Part model, mm, in its own coordinate system. Face numbers are marked on the shaded views. A direction names the side the tool comes from. Give positions to 0.01 mm unless a question says otherwise; leave off trailing zeros. Order: outer loops, then holes, each group sorted by start corner. A loop starts at its lowest first (then second) coordinate and runs counter-clockwise, first axis right, second up.
1. Drop flat-ended pins along their axis: pin 1 Ø5 at (y, z) = (8, 11) entering from +X; pin 2 Ø10 at (x, z) = (7.5, 12) entering from -Y; pin 3 Ø8 at (x, z) = (7.5, 10.5) entering from -Y. Give the stop position or say it passes through.
2. Probe line 1 (Y direction, x = 0, z = 0.65); line 2 (X direction, y = -8, z = 1). List the from-to ranges inside material, lowest first.
3. Mould opens along X. For the marked faces 3, 4 and 5 say: +X half, -X half, draft (parallel to the pull), parting line (faces both ways), or undercut.
4. Which spindle directions (+Z, -Z, +X, -X, +Y, -Y) get a long thin tool onto all of the face, cutting with end or side? Do the marked faces 1 and 2. Say none if no direction does.
5. Slice it at D-D on y = 0. List the corners of the cut face in (x, z).
6. Slice it at A-A on y = 8. List the corners of the cut face in (x, z), and give its area (3 significant figures).
7. Slice it at B-B on z = 23.75. List the corners of the cut face in (x, y).
from build123d import *

# Parameters (mm, degrees)
F0_R     = 10
F0_R_2   = 6
F1_DEPTH = 2
F0_R_3   = 3.5
F2_DEPTH = 25
F4_DEPTH = 20
F5_D     = 3.2


with BuildPart() as f1:
    # F0 (on Top) → F1 (new body)
    with BuildSketch(Plane.XY):
        Circle(F0_R)
        Circle(F0_R_2, mode=Mode.SUBTRACT)
    extrude(amount=F1_DEPTH)

    # F0 (on Top) → F2 (join)
    with BuildSketch(Plane.XY):
        Circle(F0_R_2)
        Circle(F0_R_3, mode=Mode.SUBTRACT)
    extrude(amount=F2_DEPTH)

    # F3 (on face) → F4 (cut)
    with BuildSketch(Plane.XY.offset(25)):
        Polygon((1.361971, -4.292439), (4.398347, -0.966719), (3.036376, 3.325721), (-1.361971, 4.292439), (-4.398347, 0.966719), (-3.036376, -3.325721), align=None)
    extrude(amount=-F4_DEPTH, mode=Mode.SUBTRACT)

    # F5 (through all)
    with Locations(Plane(origin=(0, 0, 0), x_dir=(1, 0, 0), z_dir=(0, 0, -1))):
        with Locations((-8, 0), (0, 8), (8, 0), (0, -8)):
            Hole(F5_D / 2)


solid = f1.part
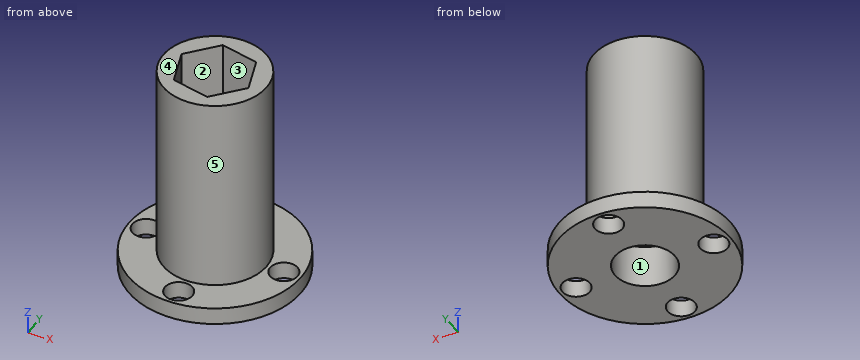
Data:
1. pin 1: stops at x = 2.4
1. pin 2: stops at y = -5.45
1. pin 3: stops at y = -4.87
2. line 1: y = -10 to -9.6, -6.4 to -3.5, 3.5 to 6.4, 9.6 to 10
2. line 2: x = -6 to -1.6, 1.6 to 6
3. face 3: undercut
3. face 4: draft
3. face 5: parting line
4. face 1: +Z, -Z
4. face 2: +Z
5. outline: (-10, 0) - (-9.6, 0) - (-9.6, 2) - (-10, 2) - close; (-6.4, 0) - (-3.5, 0) - (-3.5, 5) - (-4.09, 5) - (-4.09, 25) - (-6, 25) - (-6, 2) - (-6.4, 2) - close; (3.5, 0) - (6.4, 0) - (6.4, 2) - (6, 2) - (6, 25) - (4.09, 25) - (4.09, 5) - (3.5, 5) - close; (9.6, 0) - (10, 0) - (10, 2) - (9.6, 2) - close
6. outline: (-6, 0) - (-1.6, 0) - (-1.6, 2) - (-6, 2) - close; (1.6, 0) - (6, 0) - (6, 2) - (1.6, 2) - close
6. area: 17.6 mm2
7. outline: circle Ø12 at (0, 0); hole (-4.4, 0.97) - (-3.04, -3.33) - (1.36, -4.29) - (4.4, -0.97) - (3.04, 3.33) - (-1.36, 4.29) - close
